```python
from build123d import *

# Parameters (mm, degrees)
F0_W     = 1900
F0_H     = 1800
F1_DEPTH = 250
F2_T     = -2
F4_D     = 300
F4_DEPTH = 1200.001


with BuildPart() as f1:
    # F0 (on Front) → F1 (new body, symmetric)
    with BuildSketch(Plane.XZ):
        Rectangle(F0_W, F0_H)
        Polygon((-950, 900), (950, 900), (175, 1200), (0, 1200), (-175, 1200), align=None)
    extrude(amount=F1_DEPTH, both=True)

    # F2
    f2_openings = [f1.faces().sort_by_distance(p)[0] for p in [
        (0, -250, 91.217565),
    ]]
    offset(amount=F2_T, openings=f2_openings)

    # F4 (through all, one way)
    with BuildSketch(Plane(origin=(0, 0, 0), x_dir=(1, 0, 0), z_dir=(0, 0, -1))):
        with Locations((0, 0)):
            Circle(F4_D / 2)
    extrude(amount=-F4_DEPTH, mode=Mode.SUBTRACT)


solid = f1.part
```
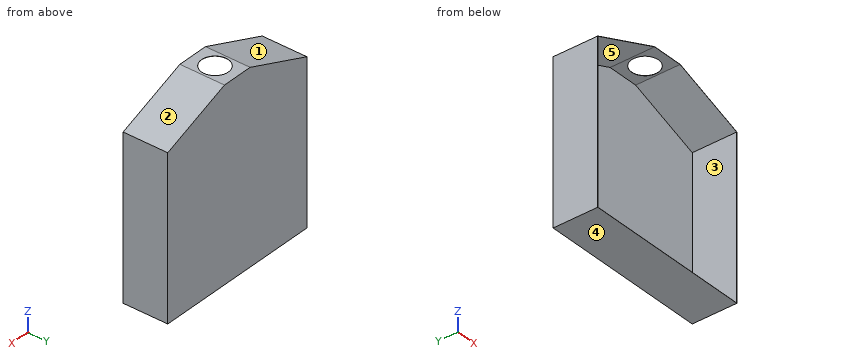
The model under review builds one solid part; all positions refer to its coordinate system, in mm. Face numbers are marked on the shaded views. A direction names the side the tool comes from. Round coordinates to 2 decimals unless told otherwise and drop trailing zeros. Loops run counter-clockwise (first coordinate to the right, second up) from the corner with the lowest first, then second, coordinate; pieces in that order, holes last.
Item 1: Take a section at C-C (y = 0). Write out the cut boundary in (x, z).
Determined:
outline: (-950, -900) - (950, -900) - (950, 900) - (175, 1200) - (150, 1200) - (150, 1198) - (174.63, 1198) - (948, 898.63) - (948, -898) - (-948, -898) - (-948, 898.63) - (-174.63, 1198) - (-150, 1198) - (-150, 1200) - (-175, 1200) - (-950, 900) - close
Item 2: For line 1 (X direction, y = -116.5, z = 889.5); line 2 (Y direction, x = 0, z = 1198.85); line 3 (Y direction, x = 760, z = 354), list the stretches that pass through material, from the lowest coordinate up.
Determined:
line 1: x = -950 to -948, 948 to 950
line 2: y = -250 to -150, 150 to 250
line 3: y = 248 to 250
Item 3: Mouldability with a two-part tool opening along X and no side actions: class the marked faces 1, 2 and 3 as released by +X, released by -X, zero draft, split by the parting line, or undercut.
Determined:
face 1: released by -X
face 2: released by +X
face 3: undercut
Item 4: Clearance check with a flat-ended pin moving along its axis: pin 1 Ø4 at (x, y) = (-117.5, 10) entering from +Z. State where the tip first meets the part, or that it passes through.
Determined:
pin 1: stops at z = -898
Item 5: Take a section at A-A (x = 0). Write out the cut boundary in (y, z), then the cut area to 3 significant figures.
Determined:
outline: (-250, -900) - (250, -900) - (250, 1200) - (150, 1200) - (150, 1198) - (248, 1198) - (248, -898) - (-250, -898) - close; (-250, 1198) - (-150, 1198) - (-150, 1200) - (-250, 1200) - close
area: 5,590 mm2
Item 6: For the marked faces 4 and 5, list the 3-axis set-ups (+Z, -Z, +X, -X, +Y, -Y) from which the entire face can be reached by the end or side of a thin tool; tool diameter is ignored.
Determined:
face 4: -Z, +X, -X, +Y, -Y
face 5: -Y
Item 7: Take a section at D-D (x = 282). Write out the cut boundary in (y, z).
Determined:
outline: (-250, -900) - (250, -900) - (250, 1158.58) - (-250, 1158.58) - (-250, 1156.44) - (248, 1156.44) - (248, -898) - (-250, -898) - close
Item 8: Take a section at B-B (z = 704). Write out the cut boundary in (x, y), then the cut area to 3 significant figures.
Determined:
outline: (-950, -250) - (-948, -250) - (-948, 248) - (948, 248) - (948, -250) - (950, -250) - (950, 250) - (-950, 250) - close
area: 5,790 mm2
